Geometry check sheet. Reference: drawing and pictorial views, mm from the part's lowest x, y, z. A direction names the side the tool comes from. Give positions to 0.01 mm unless a question says otherwise; leave off trailing zeros. Write each loop counter-clockwise with the first axis right and the second up, starting at its lowest first coordinate (ties: lowest second). Pieces come first, ordered by that corner, then holes. Notation, with made-up numbers: M -8,37 L 25,37 A34 ccw 25,76 Z; hole C 6.5,9 d6. An arc over 180 degrees is marked long. Write item = value, one per line. Start each with the question number.
1) Cross-section at D-D, the plane y = 8.75. Record the cut outline in (x, z), plus the area to 3 significant figures.
2) Go/stop test with flat-tipped pins: pin 1 (11.5 mm diameter, centred on x = 12.5, y = 21, fed in from +Z); pin 2 (12 mm diameter, centred on x = 12.5, z = 57.5, fed in from +Y); pin 3 (6.5 mm diameter, centred on y = 7, z = 15, fed in from -X); pin 4 (3 mm diameter, centred on y = 4.5, z = 53.5, fed in from -X). Record where each tip stops, or that it passes through.
3) Scan lines: line 1 along X through (y, z) = (22, 28.5); line 2 along Y through (x, z) = (18, 45) (3 decimals). Record each from-to range of solid material in increasing order. Write a range as [from, to].
4) Cross-section at A-A, the plane y = 13.5. Record the cut outline in (x, z), plus the area to 3 significant figures.
5) Mould release check, pull along Z, two halves, no side actions. Record for the marked faces 1, 2 and 3: released by +Z, released by -Z, zero draft, split by the parting line, or undercut.
6) Access from +Z, -Z, +X, -X, +Y, -Y to the whole of each face (thin tool, end or side, straight path). Record for the marked faces 4, 5 and 6.
7) Cross-section at C-C, the plane x = 16. Record the cut outline in (y, z) (3 decimals).
8) Cross-section at B-B, the plane z = 15. Record the cut outline in (x, y) (3 decimals).
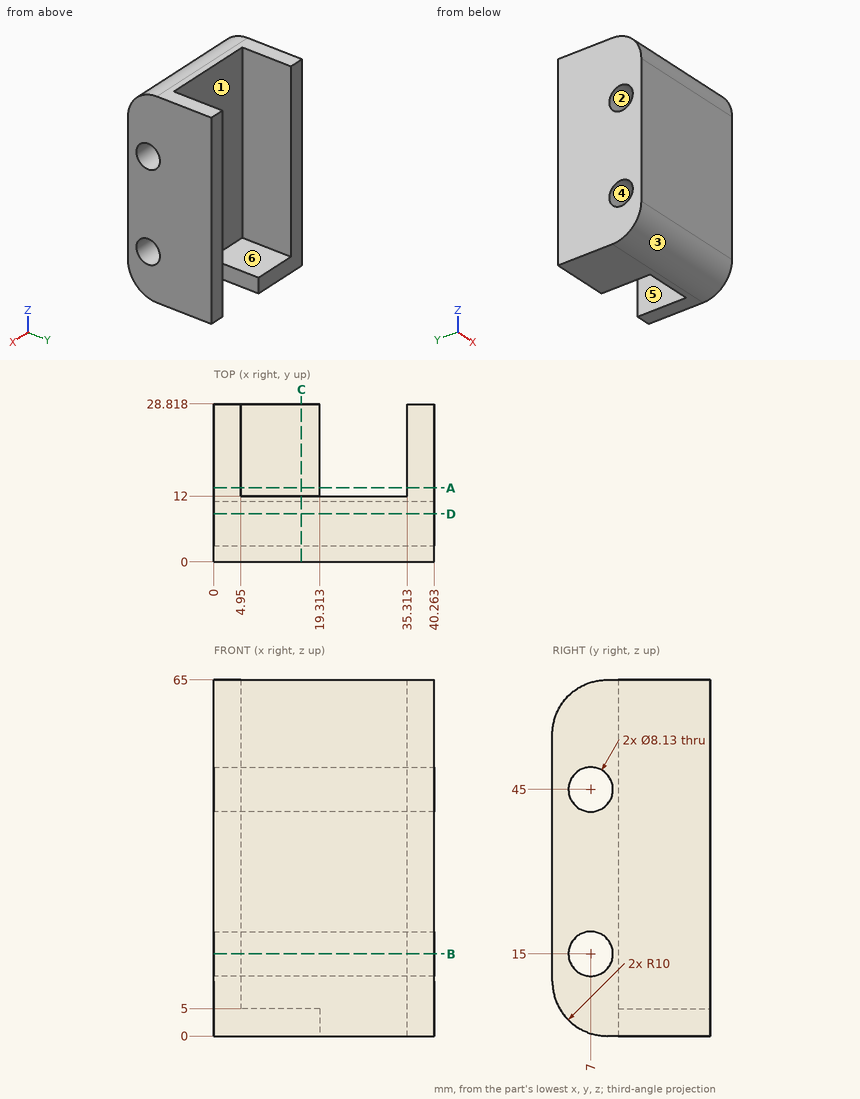
Reply:
q1.outline = M 0,0.08 L 40.26,0.08 L 40.26,11.33 L 0,11.33 Z; M 0,18.67 L 40.26,18.67 L 40.26,41.33 L 0,41.33 Z; M 0,48.67 L 40.26,48.67 L 40.26,64.92 L 0,64.92 Z
q1.area = 2,020 mm2
q2.pin_1 = 5
q2.pin_2 = 12
q2.pin_3 = through
q2.pin_4 = 0
q3.line_1 = [0, 4.95], [35.31, 40.26]
q3.line_2 = [0, 2.935], [11.065, 12]
q4.outline = M 0,0 L 19.31,0 L 19.31,5 L 4.95,5 L 4.95,65 L 0,65 Z; M 35.31,0 L 40.26,0 L 40.26,65 L 35.31,65 Z
q4.area = 715 mm2
q5.face_1 = zero draft
q5.face_2 = undercut
q5.face_3 = released by -Z
q6.face_4 = +X, -X
q6.face_5 = +Z, -Z, +Y
q6.face_6 = +Z, +Y
q7.outline = M 0,10 A10 ccw 10,0 L 28.818,0 L 28.818,5 L 12,5 L 12,65 L 10,65 A10 ccw 0,55 Z; hole C 7,15 d8.13; hole C 7,45 d8.13
q8.outline = M 0,0 L 40.263,0 L 40.263,2.935 L 0,2.935 Z; M 0,11.065 L 40.263,11.065 L 40.263,28.818 L 35.313,28.818 L 35.313,12 L 4.95,12 L 4.95,28.818 L 0,28.818 Z
